Part model, mm, in its own coordinate system. Coordinates: 2 decimals unless noted, no trailing zeros. Loops run counter-clockwise (first coordinate to the right, second up) from the corner with the lowest first, then second, coordinate; pieces in that order, holes last. Notation, with made-up numbers: (-30, -35.5) - (-17, -35.5) arc R8 cw to (-17, -24.5) - close; hole circle Ø1 at (12.25, 43.5). An arc over 180 degrees is marked (long way). Use a Markdown table: item, result. Add a question column.
1) Band-saw the part on A-A (x = -12.7). Give the cut face in (y, z), plus the area to 3 significant figures.
2) Probe probe 1 along X at (y, z) = (602, -131). List the from-to ranges inside material, lowest first. Write a range as [from, to].
3) Band-saw the part on C-C (z = -48). Give the cut face in (x, y), plus the area to 3 significant figures.
4) Band-saw the part on D-D (x = 433). Give the cut face in (y, z), plus the area to 3 significant figures.
5) Band-saw the part on B-B (y = 304). Give the cut face in (x, z).
6) Drop flat-ended pins along their axis: P1, Ø14, axis at y = 294.5, z = -132.5, coming from the +X side; P2, Ø4, axis at x = 422, z = -131.5, coming from the -Y side; P3, Ø7.5, axis at x = -27.5, z = -132.5, coming from the -Y side. Give the stop position or say it passes through.
from build123d import *

# Parameters (mm, degrees)
F0_R     = 12.7
F1_DEPTH = 254
F2_W     = 711.2
F2_H     = 12.7
F3_DEPTH = 32.258
F4_W     = 609.6
F4_H     = 12.7
F5_DEPTH = 25.4


with BuildPart() as f1:
    # F0 (on Top) → F1 (new body)
    with BuildSketch(Plane.XY):
        with Locations((-12.7, 44.464361)):
            Circle(F0_R)
    extrude(amount=-F1_DEPTH)

    # F2 (on Right) → F3 (join)
    with BuildSketch(Plane.YZ):
        with Locations((401.540584, -133.65126)):
            Rectangle(F2_W, F2_H)
    extrude(amount=-F3_DEPTH)

    # F4 (on face) → F5 (join)
    with BuildSketch(Plane(origin=(0, 757.140584, 0), x_dir=(-1, 0, 0), z_dir=(0, 1, 0))):
        with Locations((-272.542, -133.65126)):
            Rectangle(F4_W, F4_H)
    extrude(amount=F5_DEPTH)


solid = f1.part
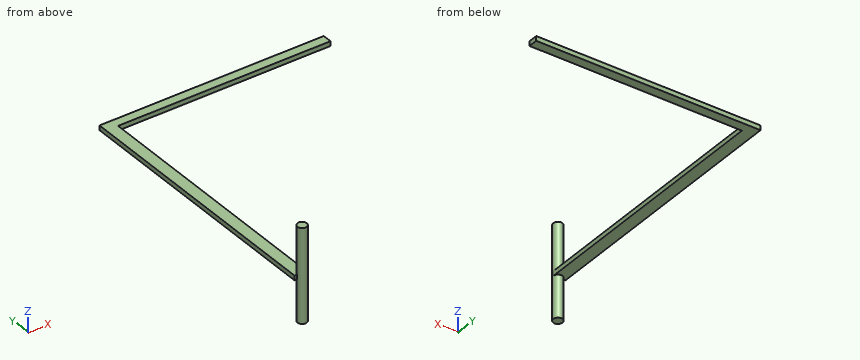
Answer block:
| question | item | result |
|---|---|---|
| 1 | outline | (31.76, -254) - (57.16, -254) - (57.16, -140) - (782.54, -140) - (782.54, -127.3) - (57.16, -127.3) - (57.16, 0) - (31.76, 0) - close |
| 1 | area | 15,700 mm2 |
| 2 | probe 1 | [-32.26, 0] |
| 3 | outline | circle Ø25.4 at (-12.7, 44.46) |
| 3 | area | 507 mm2 |
| 4 | outline | (757.14, -140) - (782.54, -140) - (782.54, -127.3) - (757.14, -127.3) - close |
| 4 | area | 323 mm2 |
| 5 | outline | (-32.26, -140) - (0, -140) - (0, -127.3) - (-32.26, -127.3) - close |
| 6 | P1 | x = 0 |
| 6 | P2 | y = 757.14 |
| 6 | P3 | y = 38.2 |
